Could you check a few things on this model? Use its own coordinates, in mm. A direction names the side the tool comes from. Round coordinates to 2 decimals unless told otherwise and drop trailing zeros. Write each loop counter-clockwise with the first axis right and the second up, starting at its lowest first coordinate (ties: lowest second). Pieces come first, ordered by that corner, then holes. Notation, with made-up numbers: M 79.5,-7 L 88.5,-7 A28 cw 88.5,28 Z; hole C 56,24 d2. An arc over 180 degrees is marked long. One line per item, written item: value. Start each with the question number.
(1) I want a section at A-A on y = 0. Please give me the cut outline in (x, z).
(2) If I drill on L1, parallel to Z at x = 5, y = -6.5; L2, parallel to X at y = 0.5, z = 5.5; L3, parallel to Z at x = 3.5, y = -4, over which ranges is the centre line in solid material (lowest first)?
(3) Thinking about a two-plate mould opening in Z: for faces 6 (the face through (-6, -4, 23.6)), 7 (the face through (-12, 5, 5)), 8 (the face through (-4.6, -6.2, 12.85)), which applies, released by +Z, released by -Z, zero draft, split by the parting line, or undercut?
(4) I want a section at C-C on x = 9.75. Please give me the cut outline in (y, z).
(5) I want a section at B-B on z = 6.5. Please give me the cut outline in (x, y), and give its area (3 significant figures).
(6) Which directions (+Z, -Z, +X, -X, +Y, -Y) give clear straight access to the entire face, cutting with the end or side of a thin tool? Please do faces 1 (the face through (12, -6, 5)), 2 (the face through (-8, -6, 18.85)), 3 (the face through (11.5, -3.25, -1.6)), 4 (the face through (-10.296, -4.324, 13.466)), 5 (the face through (-11.5, -6.7, -1.6)).
(7) I want a section at D-D on z = 20.75. Please give me the cut outline in (x, y).
(8) I'm going to push flat-ended pins straight in: pin 1 Ø7.5 at (y, z) = (5.5, 4) entering from -X; pin 2 Ø1.6 at (y, z) = (6, -2) entering from -X; pin 3 Ø7.5 at (y, z) = (4, 3.5) entering from +X; pin 4 Ø8 at (y, z) = (3, 10.5) entering from -X. Where does each tip first touch, or does it pass through?
```python
from build123d import *

# Parameters (mm, degrees)
F0_W      = 24
F0_H      = 18
F1_DEPTH  = 10.25
F2_R      = 2
F3_DEPTH  = 2.6
F4_R      = 4
F4_R_2    = 2
F5_DEPTH  = 1.25
F6_R      = 2
F7_DEPTH  = 4.75
F8_R      = 2.6
F9_DEPTH  = 4.75
F10_R     = 2
F11_DEPTH = 10.25
F12_R     = 1.45
F13_DEPTH = 25
F14_W     = 1
F14_H     = 1.5
F15_DEPTH = 3.3


with BuildPart() as f1:
    # F0 (on Top) → F1 (new body)
    with BuildSketch(Plane.XY):
        Rectangle(F0_W, F0_H)
    extrude(amount=F1_DEPTH)

    # F2 (on face) → F3 (join)
    with BuildSketch(Plane.XY.offset(10.25)):
        with Locations((-6.3, -4.5)):
            Circle(F2_R)
        with Locations((6.3, -4.5)):
            Circle(F2_R)
    extrude(amount=F3_DEPTH)

    # F4 (on face) → F5 (join)
    with BuildSketch(Plane.XY.offset(12.85)):
        with Locations((-6.3, -4.5)):
            Circle(F4_R)
        with Locations((-6.3, -4.5)):
            Circle(F4_R_2, mode=Mode.SUBTRACT)
        with Locations((6.3, -4.5)):
            Circle(F4_R)
        with Locations((-6.3, -4.5)):
            Circle(F4_R_2)
    extrude(amount=F5_DEPTH)

    # F6 (on face) → F7 (join)
    with BuildSketch(Plane.XY.offset(14.1)):
        with Locations((6.3, -4.5)):
            Circle(F6_R)
        with Locations((-6.3, -4.5)):
            Circle(F6_R)
    extrude(amount=F7_DEPTH)

    # F8 (on face) → F9 (join)
    with BuildSketch(Plane.XY.offset(18.85)):
        with Locations((-6.3, -4.5)):
            Circle(F8_R)
        with Locations((6.3, -4.5)):
            Circle(F8_R)
    extrude(amount=F9_DEPTH)

    # F10 (on face) → F11 (join)
    with BuildSketch(Plane.XY.offset(10.25)):
        with Locations((-12, 0)):
            Circle(F10_R)
        with Locations((12, 0)):
            Circle(F10_R)
    extrude(amount=-F11_DEPTH)

    # F12 (on face) → F13 (cut)
    with BuildSketch(Plane.XY.offset(10.25)):
        with Locations((-12, 0)):
            Circle(F12_R)
        with Locations((12, 0)):
            Circle(F12_R)
    extrude(amount=-F13_DEPTH, mode=Mode.SUBTRACT)

    # F14 (on face) → F15 (join)
    with BuildSketch(Plane(origin=(0, 0, 0), x_dir=(1, 0, 0), z_dir=(0, 0, -1))):
        with Locations((-11.5, 5.95)):
            Rectangle(F14_W, F14_H)
        with Locations((-11.5, -5.95)):
            Rectangle(F14_W, F14_H)
        with Locations((11.5, -5.95)):
            Rectangle(F14_W, F14_H)
        with Locations((11.5, 4)):
            Rectangle(F14_W, F14_H)
    extrude(amount=F15_DEPTH)


solid = f1.part
```
Found:
1. outline: M -14,0 L -13.45,0 L -13.45,10.25 L -14,10.25 Z; M -10.55,0 L 10.55,0 L 10.55,10.25 L -10.55,10.25 Z; M 13.45,0 L 14,0 L 14,10.25 L 13.45,10.25 Z
2. L1: z = 0 to 10.25, 12.85 to 14.1, 18.85 to 23.6
2. L2: x = -13.94 to -13.36, -10.64 to 10.64, 13.36 to 13.94
2. L3: z = 0 to 10.25, 12.85 to 14.1
3. face 6: released by +Z
3. face 7: zero draft
3. face 8: undercut
4. outline: M -9,0 L 9,0 L 9,10.25 L -9,10.25 Z; M -6.52,12.85 L -2.48,12.85 L -2.48,14.1 L -6.52,14.1 Z
5. outline: M -12,-9 L 12,-9 L 12,-2 A2 ccw 12,2 L 12,9 L -12,9 L -12,2 A2 ccw -12,-2 Z; hole C -12,0 d2.9; hole C 12,0 d2.9
5. area: 431 mm²
6. face 1: +Z, -Z, +X, -Y
6. face 2: none
6. face 3: -Z, +X, -X
6. face 4: +Z
6. face 5: -Z, +X, -X, -Y
7. outline: C -6.3,-4.5 d5.2; C 6.3,-4.5 d5.2
8. pin 1: stops at x = -12.97
8. pin 2: stops at x = -12
8. pin 3: stops at x = 13.98
8. pin 4: stops at x = -14
